Geometry: final body of the model. Coordinates: model frame, mm. A direction names the side the tool comes from. Round coordinates to 2 decimals unless told otherwise and drop trailing zeros. Loops run counter-clockwise (first coordinate to the right, second up) from the corner with the lowest first, then second, coordinate; pieces in that order, holes last. Notation, with made-up numbers: (39, 87) - (78, 87) arc R10 cw to (78, 94) - close; hole circle Ø9 at (5.5, 40.5). An arc over 180 degrees is marked (long way). Answer as CSV lines item,"result".
Autodesk Fusion 360 part; units mm, degrees
sketch "Sketch1" plane through (0, 0, 0) normal (0, 0, 1) x (1, 0, 0)
  line L0 (55, -3) -> (4, -3)
  line L1 (-55, -3) -> (-55, 3)
  line L2 (4, 3) -> (55, 3)
  line L3 (55, 3) -> (55, -3)
  arc A0 (4, 3) -> (4, -3) centre (0, 0) ccw
  dimension "d1" = 10
  dimension "d3" = 6
extrude "Extrude1" add sketch "Sketch1" along normal blind 3
sketch "Sketch2" plane through (0, 0, 3) normal (0, 0, 1) x (-1, 0, 0)
  line L0 (-55, -3) -> (-4, -3)
  arc A0 (-4, -3) -> (-4, 3) centre (0, 0) ccw
  line L1 (-4, 3) -> (-55, 3)
  line L2 (-55, 3) -> (-55, -3)
  circle A1 centre (0, 0) radius 1.75
  dimension "d8" = 3.5
extrude "Extrude2" cut sketch "Sketch2" against normal blind 3 contours A1
sketch "Sketch3" plane through (0, 0, 3) normal (0, 0, 1) x (-1, 0, 0)
  circle A0 centre (0, 0) radius 1.75
  line L0 (-55, -3) -> (-4, -3)
  arc A1 (-4, -3) -> (-4, 3) centre (0, 0) ccw
  line L1 (-4, 3) -> (-55, 3)
  line L2 (-55, 3) -> (-55, -3)
  line L3 (-55, -3) -> (-45, -3)
  line L4 (-45, -3) -> (-45, 3)
  line L5 (-45, 3) -> (-55, 3)
  line L6 (-55, 3) -> (-55, -3)
  dimension "d11" = 10
extrude "Extrude3" add sketch "Sketch3" along normal blind 25 contours L0 L1 L2 L3 L4 L5 L6
sketch "Sketch4" plane through (0, 0, 28) normal (0, 0, 1) x (-1, 0, 0)
  line L0 (-55, 3) -> (-55, -3)
  line L1 (-55, -3) -> (-45, -3)
  line L2 (-45, -3) -> (-45, 3)
  line L3 (-45, 3) -> (-55, 3)
  line L4 (-45, -3) -> (-46, -3)
  line L5 (-46, -3) -> (-46, 1.6)
  line L6 (-46, 1.6) -> (-45, 1.6)
  line L7 (-45, 1.6) -> (-45, -3)
  line L8 (-55, -3) -> (-54, -3)
  line L9 (-54, -3) -> (-54, 1.6)
  line L10 (-54, 1.6) -> (-55, 1.6)
  line L11 (-55, 1.6) -> (-55, -3)
  dimension "d14" = 4.6
  dimension "d15" = 1
extrude "Extrude4" cut sketch "Sketch4" against normal blind 6 contours L0 L1 L2 L3 L5 L6 L9 L10
(1) Material intervals for line 1 along X through (y, z) = (0, 1.15); line 2 along Y through (x, z) = (0, 1.9); line 3 along X through (y, z) = (2.25, 25), sorted ascending.
Findings below:
line 1,"-5 to -1.75, 1.75 to 55"
line 2,"-5 to -1.75, 1.75 to 5"
line 3,"45 to 46, 54 to 55"
(2) Access query for faces 1 (the face through (55, 0, 14)), 2 (the face through (47, 3, 9)), 3 (the face through (45, 0, 15)), 4 (the face through (54, 1, 25)). Directions: +Z, -Z, +X, -X, +Y, -Y. A direction counts if a zero-diameter tool reaches every point of the face in a straight line with its end or side. Return the directions, or none.
Findings below:
face 1,"+Z, -Z, +X, +Y, -Y"
face 2,"+Z, -Z, +X, +Y"
face 3,"+Z, -X, +Y, -Y"
face 4,"+Z, +Y, -Y"
(3) Section B-B (y = 0). Output: boundary loops of the cut face in (x, z).
Findings below:
outline,"(-5, 0) - (-1.75, 0) - (-1.75, 3) - (-5, 3) - close; (1.75, 0) - (55, 0) - (55, 28) - (54, 28) - (54, 22) - (46, 22) - (46, 28) - (45, 28) - (45, 3) - (1.75, 3) - close"
(4) Section C-C (z = 7.5). Output: boundary loops of the cut face in (x, y).
Findings below:
outline,"(45, -3) - (55, -3) - (55, 3) - (45, 3) - close"
(5) Section D-D (x = 38.5). Output: boundary loops of the cut face in (y, z), and give its area (3 significant figures).
Findings below:
outline,"(-3, 0) - (3, 0) - (3, 3) - (-3, 3) - close"
area,"18.0 mm2"
(6) Draft query along Y for faces 5 (the face through (38.8, -3, 2.8)), 6 (the face through (-5, 0, 1)), 7 (the face through (25, 0, 0)), 8 (the face through (-1.617, 0.67, 1.521)). Return one class per face: pulls with the +Y half, pulls with the -Y half, needs draft (parallel to the pull), parting line crosses it, or undercut.
Findings below:
face 5,"pulls with the -Y half"
face 6,"parting line crosses it"
face 7,"needs draft"
face 8,"undercut"
(7) Section A-A (x = 0). Output: boundary loops of the cut face in (y, z).
Findings below:
outline,"(-5, 0) - (-1.75, 0) - (-1.75, 3) - (-5, 3) - close; (1.75, 0) - (5, 0) - (5, 3) - (1.75, 3) - close"
(8) Pin query (flat end, axial travel): P1, Ø2, axis at x = 0, y = 0, coming from the -Z side; P2, Ø5, axis at y = 0.5, z = 8.5, coming from the -X side; P3, Ø0.5, axis at x = 45.5, z = 24, coming from the -Y side. Return the tip coordinate at first contact, or that it passes through.
Findings below:
P1,"through"
P2,"x = 45"
P3,"y = -1.6"
